The listing builds one solid part. Answer for the finished solid, in the listing's coordinates (mm). A direction names the side the tool comes from. Coordinates: 2 decimals unless noted, no trailing zeros. Loops run counter-clockwise (first coordinate to the right, second up) from the corner with the lowest first, then second, coordinate; pieces in that order, holes last. Notation, with made-up numbers: M -26,56.5 L 30,56.5 A23 ccw 30,72.5 Z; hole C -36.5,2.5 d1. An arc over 180 degrees is marked long. Return JSON: item names as keys, results as strings. Group by question number.
1. Given P1, Ø1.6, axis at x = -33, y = 1.5, coming from the -Z side; P2, Ø1.6, axis at y = 1, z = -37.5, coming from the +X side; P3, Ø1.6, axis at x = 51, y = 2, coming from the +Z side, each flat-ended and moving along its own axis, determine where each tip first touches the part or whether it passes through.
2. Section C-C (y = 2.15) is taken. Count the separate pieces of the cut face and the enclosed holes in it, then the cut area to 3 significant figures.
3. Straight lines are drawn through the part: L1, parallel to X at y = 2.2, z = 0; L2, parallel to X at y = 0.45, z = 68; L3, parallel to Z at x = 28, y = 2.8. For each, find the intervals that lie inside material, in ascending order. Write a range as from..to.
4. Which of the six approach directions +Z, -Z, +X, -X, +Y, -Y give full straight-line access (tool end or side, diameter ignored) to faces 4 (the face through (-50.1, 1.6, 51.5)), 5 (the face through (-77.954, 1.61, -6.129))?
5. The mould has two halves that part along X. Classify faces 1 (the face through (-46.82, 1.61, 45.8)), 2 (the face through (-51.5, 1.6, -50.1)), 3 (the face through (51.5, 1.6, 50.1)): pulls with the +X half, pulls with the -X half, needs draft (parallel to the pull), parting line crosses it, or undercut.
6. Section B-B (z = -57.5) is taken. Write down the section's boundary in (x, y) (1 decimal), then the cut area to 3 significant figures.
7. Section A-A (x = -75.5) is taken. Write down the section's boundary in (y, z) (3 decimals), then the cut area to 3 significant figures.
```python
from build123d import *

# Parameters (mm, degrees)
SKETCH1_R           = 2
BOSS_EXTRUDE1_DEPTH = 3.175
CUT_EXTRUDE1_DEPTH  = 144.719172782
FILLET1_R           = 12.7
FILLET2_R           = 3.175


with BuildPart() as part:
    # Sketch1 → Boss-Extrude1 (new body)
    with BuildSketch(Plane(origin=(0, 0, 0), x_dir=(1, 0, 0), z_dir=(0, 1, 0))):
        Polygon((0, -101.6), (-101.6, 0), (0, 101.6), (101.6, 0), align=None)
        with Locations(Location((0, 82.731493173, 0), (0, 0, 270))):
            Circle(SKETCH1_R, mode=Mode.SUBTRACT)
        with Locations(Location((-82.731493173, 0, 0), (0, 0, 270))):
            Circle(SKETCH1_R, mode=Mode.SUBTRACT)
        with Locations(Location((0, -82.731493173, 0), (0, 0, 270))):
            Circle(SKETCH1_R, mode=Mode.SUBTRACT)
        with Locations(Location((82.731493173, 0, 0), (0, 0, 270))):
            Circle(SKETCH1_R, mode=Mode.SUBTRACT)
    extrude(amount=BOSS_EXTRUDE1_DEPTH)

    # Sketch2 → Cut-Extrude1 (cut, through all)
    with BuildSketch(Plane(origin=(0, 3.175, 0), x_dir=(1, 0, 0), z_dir=(0, 1, 0))):
        Polygon((-4.7625, -4.7625), (-82.55, -4.7625), (-82.55, -10.069743879), (-10.069743879, -82.55), (-4.7625, -82.55), align=None)
        Polygon((-4.7625, 4.7625), (-4.7625, 82.55), (-10.069743879, 82.55), (-82.55, 10.069743879), (-82.55, 4.7625), align=None)
        Polygon((4.7625, 82.55), (4.7625, 4.7625), (82.55, 4.7625), (82.55, 10.069743879), (10.069743879, 82.55), align=None)
        Polygon((4.7625, -4.7625), (4.7625, -82.55), (10.069743879, -82.55), (82.55, -10.069743879), (82.55, -4.7625), align=None)
    extrude(amount=-CUT_EXTRUDE1_DEPTH, mode=Mode.SUBTRACT)

    # Fillet1
    # the kernel refuses this fillet: 12.7 mm, written as the material it adds along each edge
    with BuildSketch(Plane(origin=(4.7625, 3.175, 82.55), x_dir=(0, 0, -1), z_dir=(0, -1, 0)), Plane(origin=(-82.55, 3.175, 4.7625), x_dir=(1, 0, 0), z_dir=(0, -1, 0)), Plane(origin=(-4.7625, 3.175, -82.55), x_dir=(0, 0, 1), z_dir=(0, -1, 0))) as fillet1_piece_1:
        with BuildLine():
            CenterArc((10.326526857, 12.7), FILLET1_R, 215.59885924, 54.40114076)
            Line((0, 5.307243879), (-0.206530537, 5.159388757))
            ThreePointArc((-0.206530537, 5.159388757), (-0.254, 2.653621939), (-0.254, 0))
            Line((-0.254, 0), (0, -0.254))
            Line((0, -0.254), (10.326526857, -0.254))
            Line((10.326526857, -0.254), (10.326526857, 0))
        make_face()
    extrude(amount=3.175)
    with BuildSketch(Plane(origin=(4.7625, 3.175, 4.7625), x_dir=(0, 0, 1), z_dir=(0, -1, 0)), Plane(origin=(-4.7625, 3.175, -4.7625), x_dir=(0, 0, -1), z_dir=(0, -1, 0)), Plane(origin=(-4.7625, 3.175, 4.7625), x_dir=(-1, 0, 0), z_dir=(0, -1, 0))) as fillet1_piece_2:
        with BuildLine():
            CenterArc((FILLET1_R, -FILLET1_R), FILLET1_R, 90, 90)
            Line((0, -FILLET1_R), (-FILLET1_R * 0.02, -FILLET1_R))
            Line((-FILLET1_R * 0.02, -FILLET1_R), (-FILLET1_R * 0.02, FILLET1_R * 0.02))
            Line((-FILLET1_R * 0.02, FILLET1_R * 0.02), (FILLET1_R, FILLET1_R * 0.02))
            Line((FILLET1_R, FILLET1_R * 0.02), (FILLET1_R, 0))
        make_face()
    extrude(amount=3.175)
    with BuildSketch(Plane(origin=(82.55, 3.175, 4.7625), x_dir=(-1, 0, 0), z_dir=(0, -1, 0)), Plane(origin=(-4.7625, 3.175, 82.55), x_dir=(0, 0, -1), z_dir=(0, -1, 0)), Plane(origin=(-82.55, 3.175, -4.7625), x_dir=(1, 0, 0), z_dir=(0, -1, 0)), Plane(origin=(4.7625, 3.175, -82.55), x_dir=(0, 0, 1), z_dir=(0, -1, 0))) as fillet1_piece_3:
        with BuildLine():
            CenterArc((10.326526857, -12.7), FILLET1_R, 90, 54.40114076)
            Line((0, -5.307243879), (-0.206530537, -5.159388757))
            ThreePointArc((-0.206530537, -5.159388757), (-0.254, -2.653621939), (-0.254, 0))
            Line((-0.254, 0), (0, 0.254))
            Line((0, 0.254), (10.326526857, 0.254))
            Line((10.326526857, 0.254), (10.326526857, 0))
        make_face()
    extrude(amount=3.175)
    with BuildSketch(Plane(origin=(82.55, 3.175, -4.7625), x_dir=(0, 0, -1), z_dir=(0, -1, 0))) as fillet1_piece_4:
        with BuildLine():
            CenterArc((12.7, -10.326526857), FILLET1_R, 125.59885924, 54.40114076)
            Line((0, -10.326526857), (-0.254, -10.326526857))
            Line((-0.254, -10.326526857), (-0.254, 0))
            Line((-0.254, 0), (0, 0.254))
            ThreePointArc((0, 0.254), (2.653621939, 0.254), (5.159388757, 0.206530537))
            Line((5.159388757, 0.206530537), (5.307243879, 0))
        make_face()
    extrude(amount=3.175)
    with BuildSketch(Plane(origin=(4.7625, 3.175, -4.7625), x_dir=(0, 0, -1), z_dir=(0, -1, 0))) as fillet1_piece_5:
        with BuildLine():
            CenterArc((FILLET1_R, FILLET1_R), FILLET1_R, 180, 90)
            Line((0, FILLET1_R), (-FILLET1_R * 0.02, FILLET1_R))
            Line((-FILLET1_R * 0.02, FILLET1_R), (-FILLET1_R * 0.02, -FILLET1_R * 0.02))
            Line((-FILLET1_R * 0.02, -FILLET1_R * 0.02), (FILLET1_R, -FILLET1_R * 0.02))
            Line((FILLET1_R, -FILLET1_R * 0.02), (FILLET1_R, 0))
        make_face()
    extrude(amount=3.175)

    # Fillet2
    fillet2_edges = [part.edges().sort_by_distance(p)[0] for p in [
        (0, 1.5875, 101.6),
        (-101.6, 1.5875, 0),
        (0, 1.5875, -101.6),
        (101.6, 1.5875, 0),
    ]]
    fillet(fillet2_edges, radius=FILLET2_R)


solid = part.part
```
Worked out:
{
 "1": {"P1": "z = -69.4", "P2": "x = 64.9", "P3": "z = 51.4"},
 "2": {"separate pieces": "1", "enclosed holes": "8", "area": "7,160 mm^2"},
 "3": {"L1": "-100.28..-84.73, -80.73..80.73, 84.73..100.28", "L2": "-33.6..-24.62, -4.76..4.76, 24.62..33.6", "L3": "-73.6..-64.62, -4.76..4.76, 64.62..73.6"},
 "4": {"face 4": "+Z, -X, +Y, -Y", "face 5": "+Y, -Y"},
 "5": {"face 1": "undercut", "face 2": "pulls with the -X half", "face 3": "pulls with the +X half"},
 "6": {"outline": "M -44.1,0 L -35.1,0 L -35.1,3.2 L -44.1,3.2 Z; M -4.8,0 L 4.8,0 L 4.8,3.2 L -4.8,3.2 Z; M 35.1,0 L 44.1,0 L 44.1,3.2 L 35.1,3.2 Z", "area": "87.3 mm^2"},
 "7": {"outline": "M 0,-26.1 L 3.175,-26.1 L 3.175,-17.12 L 0,-17.12 Z; M 0,-5.192 L 3.175,-5.192 L 3.175,5.192 L 0,5.192 Z; M 0,17.12 L 3.175,17.12 L 3.175,26.1 L 0,26.1 Z", "area": "90.0 mm^2"}
}
